Input: part model. Units: mm. Frame: model coordinates. Give positions to 0.01 mm unless a question says otherwise; leave off trailing zeros. Loops run counter-clockwise (first coordinate to the right, second up) from the corner with the lowest first, then second, coordinate; pieces in that order, holes last. Notation, with made-up numbers: (26, 57.25) - (70, 57.25) arc R27 cw to (70, 85.25) - close; hole circle Ø3 at (0, 64.25). An arc over 180 degrees is marked (long way). One line per item, written item: value.
from build123d import *

# Parameters (mm, degrees)
F0_R     = 55
F0_R_2   = 52.5
F1_DEPTH = 6
F2_DEPTH = 3


with BuildPart() as f1:
    # F0 (on Top) → F1 (new body)
    with BuildSketch(Plane.XY):
        Circle(F0_R)
        Circle(F0_R_2, mode=Mode.SUBTRACT)
        Circle(F0_R_2)
        with BuildLine():
            Line((-4, -39.7994974843), (-4, -44.821869662))
            ThreePointArc((-4, -44.821869662), (-31.8198051534, -31.8198051534), (-44.821869662, -4))
            Line((-44.821869662, -4), (-39.7994974843, -4))
            ThreePointArc((-39.7994974843, -4), (-28.2842712475, -28.2842712475), (-4, -39.7994974843))
        make_face(mode=Mode.SUBTRACT)
        with BuildLine():
            ThreePointArc((-4, -29.7321374946), (-21.2132034356, -21.2132034356), (-29.7321374946, -4))
            Line((-29.7321374946, -4), (-24.6779253585, -4))
            ThreePointArc((-24.6779253585, -4), (-17.6776695297, -17.6776695297), (-4, -24.6779253585))
            Line((-4, -24.6779253585), (-4, -29.7321374946))
        make_face(mode=Mode.SUBTRACT)
        with BuildLine():
            Line((39.7994974843, -4), (44.821869662, -4))
            ThreePointArc((44.821869662, -4), (31.8198051534, -31.8198051534), (4, -44.821869662))
            Line((4, -44.821869662), (4, -39.7994974843))
            ThreePointArc((4, -39.7994974843), (28.2842712475, -28.2842712475), (39.7994974843, -4))
        make_face(mode=Mode.SUBTRACT)
        with BuildLine():
            ThreePointArc((29.7321374946, -4), (21.2132034356, -21.2132034356), (4, -29.7321374946))
            Line((4, -29.7321374946), (4, -24.6779253585))
            ThreePointArc((4, -24.6779253585), (17.6776695297, -17.6776695297), (24.6779253585, -4))
            Line((24.6779253585, -4), (29.7321374946, -4))
        make_face(mode=Mode.SUBTRACT)
        with BuildLine():
            Line((0.7063379744, -18.6231244003), (0, -18.6231244003))
            Line((0, -18.6231244003), (-0.7063379744, -18.6231244003))
            Line((-0.7063379744, -18.6231244003), (-0.4744689504, -9.9455872551))
            add(Edge.make_bspline(
                [(-0.4744689504, -9.9455872551), (-0.4627407761, -9.8347328603), (-0.6571381819, -9.3434378505), (-1.0671400232, -9.2586101964)],
                knots=[0, 0, 0, 0, 0.9073017578, 0.9073017578, 0.9073017578, 0.9073017578], degree=3))
            Line((-1.0671400232, -9.2586101964), (-9.3420948833, -10.3767029941))
            Line((-9.3420948833, -10.3767029941), (-8.5947467014, -7.927252911))
            add(Edge.make_bspline(
                [(-8.5947467014, -7.927252911), (-8.5831601173, -7.8032519668), (-8.5160043091, -7.4144573882), (-8.8199712336, -7.0574730635)],
                knots=[0, 0, 0, 0, 0.8984670685, 0.8984670685, 0.8984670685, 0.8984670685], degree=3))
            Line((-8.8199712336, -7.0574730635), (-17.2568876296, -0.1983663387))
            Line((-17.2568876296, -0.1983663387), (-15.4789015651, 0.6534472341))
            add(Edge.make_bspline(
                [(-15.4789015651, 0.6534472341), (-15.2981067076, 0.7015652373), (-15.0379305841, 0.9150229577), (-14.9981947616, 1.1539326515), (-15.0481807068, 1.4938330278)],
                knots=[0, 0, 0, 0, 0.4670435173, 1, 1, 1, 1], degree=3))
            Line((-15.0481807068, 1.4938330278), (-16.5220610797, 6.9137872197))
            Line((-16.5220610797, 6.9137872197), (-11.80508174, 5.9227617458))
            add(Edge.make_bspline(
                [(-11.80508174, 5.9227617458), (-11.5451579913, 5.8577810414), (-11.1852632836, 5.842785351), (-10.9203411266, 6.2926532701)],
                knots=[0, 0, 0, 0, 0.9589503078, 0.9589503078, 0.9589503078, 0.9589503078], degree=3))
            Line((-10.9203411266, 6.2926532701), (-10.265532881, 8.576983586))
            Line((-10.265532881, 8.576983586), (-6.390159484, 4.2284368537))
            add(Edge.make_bspline(
                [(-6.390159484, 4.2284368537), (-6.0810563155, 3.8955565542), (-5.2899533571, 3.7433779044), (-5.0645819865, 4.4543202966), (-5.1299692132, 4.9595851451)],
                knots=[0, 0, 0, 0, 0.4924700015, 1, 1, 1, 1], degree=3))
            Line((-5.1299692132, 4.9595851451), (-6.7966869101, 13.8145368546))
            Line((-6.7966869101, 13.8145368546), (-4.387574736, 12.5758592039))
            add(Edge.make_bspline(
                [(-4.387574736, 12.5758592039), (-3.8159328979, 12.3909162357), (-3.60577018, 12.298444286), (-3.1265998259, 12.794428505)],
                knots=[0, 0, 0, 0, 1.2797774272, 1.2797774272, 1.2797774272, 1.2797774272], degree=3))
            Line((-3.1265998259, 12.794428505), (0, 18.499981612))
            Line((0, 18.499981612), (3.1265998259, 12.794428505))
            add(Edge.make_bspline(
                [(4.387574736, 12.5758592039), (3.8159328979, 12.3909162357), (3.60577018, 12.298444286), (3.1265998259, 12.794428505)],
                knots=[0, 0, 0, 0, 1.2797774272, 1.2797774272, 1.2797774272, 1.2797774272], degree=3))
            Line((4.387574736, 12.5758592039), (6.7966869101, 13.8145368546))
            Line((6.7966869101, 13.8145368546), (5.1299692132, 4.9595851451))
            add(Edge.make_bspline(
                [(6.390159484, 4.2284368537), (6.0810563155, 3.8955565542), (5.2899533571, 3.7433779044), (5.0645819865, 4.4543202966), (5.1299692132, 4.9595851451)],
                knots=[0, 0, 0, 0, 0.4924700015, 1, 1, 1, 1], degree=3))
            Line((6.390159484, 4.2284368537), (10.265532881, 8.576983586))
            Line((10.265532881, 8.576983586), (10.9203411266, 6.2926532701))
            add(Edge.make_bspline(
                [(11.80508174, 5.9227617458), (11.5451579913, 5.8577810414), (11.1852632836, 5.842785351), (10.9203411266, 6.2926532701)],
                knots=[0, 0, 0, 0, 0.9589503078, 0.9589503078, 0.9589503078, 0.9589503078], degree=3))
            Line((11.80508174, 5.9227617458), (16.5220610797, 6.9137872197))
            Line((16.5220610797, 6.9137872197), (15.0481807068, 1.4938330278))
            add(Edge.make_bspline(
                [(15.4789015651, 0.6534472341), (15.2981067076, 0.7015652373), (15.0379305841, 0.9150229577), (14.9981947616, 1.1539326515), (15.0481807068, 1.4938330278)],
                knots=[0, 0, 0, 0, 0.4670435173, 1, 1, 1, 1], degree=3))
            Line((15.4789015651, 0.6534472341), (17.2568876296, -0.1983663387))
            Line((17.2568876296, -0.1983663387), (8.8199712336, -7.0574730635))
            add(Edge.make_bspline(
                [(8.5947467014, -7.927252911), (8.5831601173, -7.8032519668), (8.5160043091, -7.4144573882), (8.8199712336, -7.0574730635)],
                knots=[0, 0, 0, 0, 0.8984670685, 0.8984670685, 0.8984670685, 0.8984670685], degree=3))
            Line((8.5947467014, -7.927252911), (9.3420948833, -10.3767029941))
            Line((9.3420948833, -10.3767029941), (1.0671400232, -9.2586101964))
            add(Edge.make_bspline(
                [(0.4744689504, -9.9455872551), (0.4627407761, -9.8347328603), (0.6571381819, -9.3434378505), (1.0671400232, -9.2586101964)],
                knots=[0, 0, 0, 0, 0.9073017578, 0.9073017578, 0.9073017578, 0.9073017578], degree=3))
            Line((0.4744689504, -9.9455872551), (0.7063379744, -18.6231244003))
        make_face(mode=Mode.SUBTRACT)
        with BuildLine():
            Line((-4, 29.7321374946), (-4, 24.6779253585))
            ThreePointArc((-4, 24.6779253585), (-17.6776695297, 17.6776695297), (-24.6779253585, 4))
            Line((-24.6779253585, 4), (-29.7321374946, 4))
            ThreePointArc((-29.7321374946, 4), (-21.2132034356, 21.2132034356), (-4, 29.7321374946))
        make_face(mode=Mode.SUBTRACT)
        with BuildLine():
            Line((-4, 44.821869662), (-4, 39.7994974843))
            ThreePointArc((-4, 39.7994974843), (-28.2842712475, 28.2842712475), (-39.7994974843, 4))
            Line((-39.7994974843, 4), (-44.821869662, 4))
            ThreePointArc((-44.821869662, 4), (-31.8198051534, 31.8198051534), (-4, 44.821869662))
        make_face(mode=Mode.SUBTRACT)
        with BuildLine():
            ThreePointArc((4, 29.7321374946), (21.2132034356, 21.2132034356), (29.7321374946, 4))
            Line((29.7321374946, 4), (24.6779253585, 4))
            ThreePointArc((24.6779253585, 4), (17.6776695297, 17.6776695297), (4, 24.6779253585))
            Line((4, 24.6779253585), (4, 29.7321374946))
        make_face(mode=Mode.SUBTRACT)
        with BuildLine():
            Line((4, 39.7994974843), (4, 44.821869662))
            ThreePointArc((4, 44.821869662), (31.8198051534, 31.8198051534), (44.821869662, 4))
            Line((44.821869662, 4), (39.7994974843, 4))
            ThreePointArc((39.7994974843, 4), (28.2842712475, 28.2842712475), (4, 39.7994974843))
        make_face(mode=Mode.SUBTRACT)
    extrude(amount=-F1_DEPTH)

    # F0 (on Top) → F2 (cut)
    with BuildSketch(Plane.XY):
        Circle(F0_R)
        Circle(F0_R_2, mode=Mode.SUBTRACT)
    extrude(amount=-F2_DEPTH, mode=Mode.SUBTRACT)


solid = f1.part
Item 1: Section A-A, the plane x = -22. Output: boundary loops of the cut face in (y, z), and give its area (3 significant figures).
Verdict:
outline: (-50.41, -6) - (-39.26, -6) - (-39.26, 0) - (-47.67, 0) - (-47.67, -3) - (-50.41, -3) - close; (-33.41, -6) - (-20.4, -6) - (-20.4, 0) - (-33.41, 0) - close; (-11.87, -6) - (11.87, -6) - (11.87, 0) - (-11.87, 0) - close; (20.4, -6) - (33.41, -6) - (33.41, 0) - (20.4, 0) - close; (39.26, -6) - (50.41, -6) - (50.41, -3) - (47.67, -3) - (47.67, 0) - (39.26, 0) - close
area: 416 mm^2
Item 2: Pin query (flat end, axial travel): P1, Ø1.5, axis at x = 43, z = -4, coming from the +Y side; P2, Ø2.5, axis at y = -26.5, z = -3.5, coming from the +X side; P3, Ø1.5, axis at x = 41.5, z = -3.5, coming from the -Y side; P4, Ø1.5, axis at x = 42.5, y = -36, coming from the -Z side. Return the tip coordinate at first contact, or that it passes through.
Verdict:
P1: stops at y = 35.21
P2: stops at x = 48.86
P3: stops at y = -36.94
P4: stops at z = -6
Item 3: Section D-D, the plane y = -34. Output: boundary loops of the cut face in (x, z).
Verdict:
outline: (-43.23, -6) - (-29.48, -6) - (-29.48, 0) - (-40, 0) - (-40, -3) - (-43.23, -3) - close; (-21.07, -6) - (21.07, -6) - (21.07, 0) - (-21.07, 0) - close; (29.48, -6) - (43.23, -6) - (43.23, -3) - (40, -3) - (40, 0) - (29.48, 0) - close
Item 4: Material intervals for L1, parallel to Y at x = -11, z = -1.25; L2, parallel to X at y = -15, z = -2.5; L3, parallel to X at y = 25, z = -1.75, sorted ascending.
Verdict:
L1: y = -51.33 to -43.63, -38.46 to -27.91, -22.45 to -5.29, 6.17 to 22.45, 27.91 to 38.46, 43.63 to 51.33
L2: x = -50.31 to -42.43, -37.08 to -25.98, -20 to -0.61, 0.61 to 20, 25.98 to 37.08, 42.43 to 50.31
L3: x = -46.17 to -37.42, -31.22 to -16.58, -4 to 4, 16.58 to 31.22, 37.42 to 46.17
Item 5: Section C-C, the plane x = -43. Output: boundary loops of the cut face in (y, z), and give its area (3 significant figures).
Verdict:
outline: (-34.29, -6) - (-13.27, -6) - (-13.27, 0) - (-30.12, 0) - (-30.12, -3) - (-34.29, -3) - close; (-4, -6) - (4, -6) - (4, 0) - (-4, 0) - close; (13.27, -6) - (34.29, -6) - (34.29, -3) - (30.12, -3) - (30.12, 0) - (13.27, 0) - close
area: 275 mm^2
Item 6: Draft query along Y for faces 1 (the face through (5.263, -9.825, -2.958)), 2 (the face through (-1, -11, -6)), 3 (the face through (50.076, 15.77, -1.479)). Return one class per face: pulls with the +Y half, pulls with the -Y half, needs draft (parallel to the pull), parting line crosses it, or undercut.
Verdict:
face 1: undercut
face 2: needs draft
face 3: parting line crosses it
